from build123d import *

# Parameters (mm, degrees)
SKETCH022_W            = 64
SKETCH022_H            = 64
PAD020_DEPTH           = 9
SKETCH023_R            = 1.55
POCKET003_DEPTH        = 9
SKETCH024_R            = 1.55
POCKET004_DEPTH        = 9
SKETCH025_R            = 3
POCKET005_DEPTH        = 5.5
SKETCH026_R            = 6
POCKET006_DEPTH        = 9
SKETCH030_R            = 1.55
POCKET009_DEPTH        = 9
SKETCH031_W            = 30
SKETCH031_H            = 27.227398
PAD022_DEPTH           = 9
SKETCH032_R            = 1.55
POCKET010_DEPTH        = 9
SKETCH066_W            = 16.8
SKETCH066_H            = 9
PAD040_DEPTH           = 8
PAD040_FACE8_W         = 9
PAD040_FACE8_H         = 16
PAD041_DEPTH           = 7
MIRRORED_FACE11_W      = 9
MIRRORED_FACE11_H      = 18
PAD042_DEPTH           = 7
PAD043_DEPTH           = 5.8
SKETCH068_R            = 2
POCKET027_DEPTH        = 5
LINEARPATTERN_COUNT    = 3
LINEARPATTERN_PITCH    = 6.4
SKETCH069_R            = 2
POCKET028_DEPTH        = 5
LINEARPATTERN001_COUNT = 3
LINEARPATTERN001_PITCH = 6.4
SKETCH071_W            = 10
SKETCH071_H            = 4
PAD044_DEPTH           = 5.8
SKETCH073_R            = 2
POCKET029_DEPTH        = 100
SKETCH074_W            = 11
SKETCH074_H            = 6
PAD045_DEPTH           = 50
SKETCH075_W            = 11
SKETCH075_H            = 2
POCKET030_DEPTH        = 12
SKETCH076_R            = 1.55
POCKET031_DEPTH        = 10
SKETCH083_R            = 3.25
POCKET035_DEPTH        = 3.5


with BuildPart() as part:
    # Sketch022 → Pad020 (new body)
    with BuildSketch(Plane.XZ):
        Rectangle(SKETCH022_W, SKETCH022_H)
    extrude(amount=PAD020_DEPTH)

    # Sketch023 (on Face5 of Pad020) → Pocket003 (cut)
    with BuildSketch(Plane(origin=(0, 0, 0), x_dir=(1, 0, 0), z_dir=(0, 1, 0))):
        with Locations((-9.5, 7.5)):
            Circle(SKETCH023_R)
        with Locations((-23.5, 7.5)):
            Circle(SKETCH023_R)
    extrude(amount=-POCKET003_DEPTH, mode=Mode.SUBTRACT)

    # Sketch024 (on Face4 of Pocket003) → Pocket004 (cut)
    with BuildSketch(Plane(origin=(0, 0, 0), x_dir=(1, 0, 0), z_dir=(0, 1, 0))):
        with Locations((1.4, 17.5)):
            Circle(SKETCH024_R)
        with Locations((18.9, -1.5)):
            Circle(SKETCH024_R)
    extrude(amount=-POCKET004_DEPTH, mode=Mode.SUBTRACT)

    # Sketch025 (on Face4 of Pocket004) → Pocket005 (cut)
    with BuildSketch(Plane(origin=(0, 0, 0), x_dir=(1, 0, 0), z_dir=(0, 1, 0))):
        with Locations((-23.5, 7.5)):
            Circle(SKETCH025_R)
        with Locations((-9.5, 7.5)):
            Circle(SKETCH025_R)
    extrude(amount=-POCKET005_DEPTH, mode=Mode.SUBTRACT)

    # Sketch026 (on Face4 of Pocket005) → Pocket006 (cut)
    with BuildSketch(Plane(origin=(0, 0, 0), x_dir=(1, 0, 0), z_dir=(0, 1, 0))):
        with Locations((0, -20)):
            Circle(SKETCH026_R)
        with Locations((20, 20)):
            Circle(SKETCH026_R)
        with Locations((-20, 20)):
            Circle(SKETCH026_R)
    extrude(amount=-POCKET006_DEPTH, mode=Mode.SUBTRACT)

    # Sketch030 (on Face5 of Pocket006) → Pocket009 (cut)
    with BuildSketch(Plane.XZ.offset(9)):
        with Locations((7.5, -7.5)):
            Circle(SKETCH030_R)
    extrude(amount=-POCKET009_DEPTH, mode=Mode.SUBTRACT)

    # Sketch031 (on Face5 of Pocket009) → Pad022 (join)
    with BuildSketch(Plane.XZ.offset(9)):
        with Locations((-1, 45.613699)):
            Rectangle(SKETCH031_W, SKETCH031_H)
    extrude(amount=-PAD022_DEPTH)

    # Sketch032 (on Face22 of Pad022) → Pocket010 (cut)
    with BuildSketch(Plane.XZ.offset(9)):
        with Locations((-9.5, 47.5)):
            Circle(SKETCH032_R)
        with Locations((7.5, 47.5)):
            Circle(SKETCH032_R)
    extrude(amount=-POCKET010_DEPTH, mode=Mode.SUBTRACT)

    # Sketch066 (on Face2 of Pocket010) → Pad040 (join)
    with BuildSketch(Plane(origin=(-32, 0, 0), x_dir=(0, 0, -1), z_dir=(-1, 0, 0))):
        with Locations((-30.6, 4.5)):
            Rectangle(SKETCH066_W, SKETCH066_H)
    pad040 = extrude(amount=PAD040_DEPTH)

    # Pad040 Face8 → Pad041 (add)
    with BuildSketch(Plane(origin=(-24, -4.5, 32), x_dir=(0, 1, 0), z_dir=(0, 0, 1))):
        Rectangle(PAD040_FACE8_W, PAD040_FACE8_H)
    extrude(amount=PAD041_DEPTH)

    # Mirrored: Pad040 across YZ
    add(pad040.mirror(Plane.YZ))

    # Mirrored Face11 → Pad042 (add)
    with BuildSketch(Plane(origin=(23, -4.5, 32), x_dir=(0, 1, 0), z_dir=(0, 0, 1))):
        Rectangle(MIRRORED_FACE11_W, MIRRORED_FACE11_H)
    extrude(amount=PAD042_DEPTH)

    # Sketch067 (on Face27 of Pad042) → Pad043 (join)
    with BuildSketch(Plane.XZ.offset(9)):
        Polygon((40, 39), (32, 39), (32, 22.2), (40, 22.2), (40, 24.2), (34, 24.2), (34, 37), (40, 37), align=None)
    pad043 = extrude(amount=PAD043_DEPTH)

    # Mirrored001: Pad043 across YZ
    add(pad043.mirror(Plane.YZ))

    # Sketch068 (on Face37 of Mirrored001) → Pocket027 (cut)
    with BuildSketch(Plane(origin=(-34, 0, 0), x_dir=(0, 0, -1), z_dir=(-1, 0, 0))):
        with Locations((-24.2, 11.9)):
            Circle(SKETCH068_R)
    pocket027 = extrude(amount=-POCKET027_DEPTH, mode=Mode.SUBTRACT)

    # LinearPattern: Pocket027 ×3
    with Locations(*[(0, 0, i * LINEARPATTERN_PITCH) for i in range(1, LINEARPATTERN_COUNT)]):
        add(pocket027, mode=Mode.SUBTRACT)

    # Sketch069 (on Face44 of LinearPattern) → Pocket028 (cut)
    with BuildSketch(Plane(origin=(34, 0, 0), x_dir=(0, 0, 1), z_dir=(1, 0, 0))):
        with Locations((37, 11.9)):
            Circle(SKETCH069_R)
    pocket028 = extrude(amount=-POCKET028_DEPTH, mode=Mode.SUBTRACT)

    # LinearPattern001: Pocket028 ×3
    with Locations(*[(0, 0, -i * LINEARPATTERN001_PITCH) for i in range(1, LINEARPATTERN001_COUNT)]):
        add(pocket028, mode=Mode.SUBTRACT)

    # Sketch071 (on Face35 of LinearPattern001) → Pad044 (join)
    with BuildSketch(Plane.XZ.offset(9)):
        with Locations((25, 21.7)):
            Rectangle(SKETCH071_W, SKETCH071_H)
        with Locations((25, -28.3)):
            Rectangle(SKETCH071_W, SKETCH071_H)
    pad044 = extrude(amount=PAD044_DEPTH)

    # Mirrored003: Pad044 across Sketch071 V_Axis
    add(pad044.mirror(Plane(origin=(0, -9, 0), x_dir=(0, -1, 0), z_dir=(1, 0, 0))))

    # Sketch073 (on Face49 of Mirrored003) → Pocket029 (cut)
    with BuildSketch(Plane(origin=(0, 0, 23.7), x_dir=(-1, 0, 0), z_dir=(0, 0, 1))):
        with Locations((-25, 11.9)):
            Circle(SKETCH073_R)
    pocket029 = extrude(amount=-POCKET029_DEPTH, mode=Mode.SUBTRACT)

    # Mirrored004: Pocket029 across YZ
    add(pocket029.mirror(Plane.YZ), mode=Mode.SUBTRACT)

    # Sketch074 (on Face15 of Mirrored004) → Pad045 (join)
    with BuildSketch(Plane(origin=(0, 0, -32), x_dir=(1, 0, 0), z_dir=(0, 0, -1))):
        with Locations((0, 3)):
            Rectangle(SKETCH074_W, SKETCH074_H)
    extrude(amount=PAD045_DEPTH)

    # Sketch075 (on Face41 of Pad045) → Pocket030 (cut)
    with BuildSketch(Plane(origin=(5.5, 0, 0), x_dir=(0, 0, 1), z_dir=(1, 0, 0))):
        with Locations((-74.5, 3)):
            Rectangle(SKETCH075_W, SKETCH075_H)
        with Locations((-45.5, 3)):
            Rectangle(SKETCH075_W, SKETCH075_H)
    extrude(amount=-POCKET030_DEPTH, mode=Mode.SUBTRACT)

    # Sketch076 (on Face30 of Pocket030) → Pocket031 (cut)
    with BuildSketch(Plane.XZ.offset(9)):
        with Locations((29, -12.3)):
            Circle(SKETCH076_R)
        with Locations((29, -20.3)):
            Circle(SKETCH076_R)
    extrude(amount=-POCKET031_DEPTH, mode=Mode.SUBTRACT)

    # Sketch083 (on Face32 of Pocket031) → Pocket035 (cut)
    with BuildSketch(Plane.XZ.offset(9)):
        with Locations((1.4, -17.5)):
            Circle(SKETCH083_R)
    extrude(amount=-POCKET035_DEPTH, mode=Mode.SUBTRACT)


solid = part.part
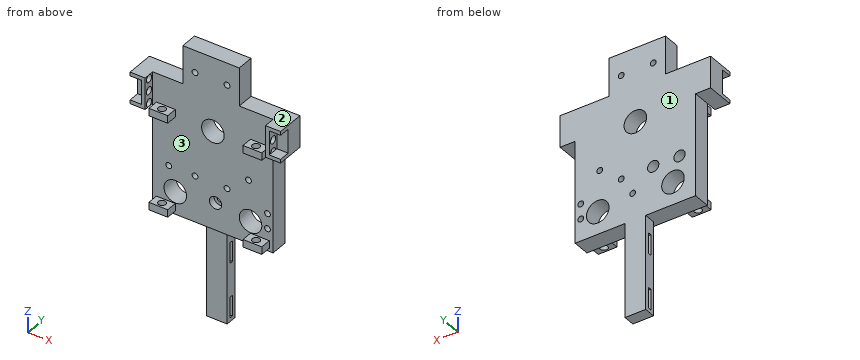
Geometry: final body of the model. Coordinates: model frame, mm. Face numbers are marked on the shaded views. Give positions to 0.01 mm unless a question says otherwise; leave off trailing zeros. Loops run counter-clockwise (first coordinate to the right, second up) from the corner with the lowest first, then second, coordinate; pieces in that order, holes last. Notation, with made-up numbers: (8.5, 57) - (65.5, 57) arc R15 cw to (65.5, 75) - close; hole circle Ø4 at (-4, -19). An arc over 180 degrees is marked (long way). One line per question, with ' | ' between items. Start each with the question number.
(1) Section query B-B on z = 47.5. Return loops of the section in (x, y), then the cut area to 3 significant figures.
(2) Section query C-C on x = 11.5. Return loops of the section in (y, z).
(3) Section query D-D on z = -49. Return loops of the section in (x, y), then the cut area to 3 significant figures.
(4) Contact query for flat-ended pins moving along their axis: pin 1 (6 mm diameter, centred on x = -26.5, z = 6.5, fed in from -Y); pin 2 (1 mm diameter, centred on y = -1.5, z = -18, fed in from -X); pin 3 (9 mm diameter, centred on x = 1.5, z = -67, fed in from -Y). Output: stop coordinate, or through.
(5) Ray query, line 1 (Z direction, x = 7, y = -0.75); line 2 (Z direction, x = -29, y = -10.5); line 3 (Z direction, x = 1.4, y = -3.1). Return the intervals inside material, ascending. Write a range as from..to.
(6) Pull-direction query (Z, two-part tool) for the marked faces 1, 2 and 3; classes: released by +Z, released by -Z, zero draft, split by the parting line, or undercut.
(7) Section query A-A on z = 1.5. Return loops of the section in (x, y), then the cut area to 3 significant figures.
The answers:
1) outline: (-16, -9) - (-11.05, -9) - (-11.05, 0) - (-16, 0) - close; (-7.95, -9) - (5.95, -9) - (5.95, 0) - (-7.95, 0) - close; (9.05, -9) - (14, -9) - (14, 0) - (9.05, 0) - close | area: 214 mm2
2) outline: (-9, -32) - (0, -32) - (0, 59.23) - (-9, 59.23) - close
3) outline: (-5.5, -6) - (5.5, -6) - (5.5, -4) - (-5.5, -4) - close; (-5.5, -2) - (5.5, -2) - (5.5, 0) - (-5.5, 0) - close | area: 44.0 mm2
4) pin 1: y = -9 | pin 2: x = -32 | pin 3: y = -6
5) line 1: -32..-8.97, -6.03..46.03, 48.97..59.23 | line 2: -30.3..-26.3, 19.7..23.7 | line 3: -82..-80, -69..-51, -40..-19.05, -15.95..14.17, 25.83..59.23
6) face 1: zero draft | face 2: released by +Z | face 3: undercut
7) outline: (-32, -9) - (17.35, -9) - (17.35, 0) - (-32, 0) - close; (20.45, -9) - (32, -9) - (32, 0) - (20.45, 0) - close | area: 548 mm2
